from build123d import *

# Parameters (mm, degrees)
SKETCH2_W           = 81.6
SKETCH2_H           = 24
SKETCH2_W_2         = 77.6
SKETCH2_H_2         = 20
BOSS_EXTRUDE1_DEPTH = 7.7
SKETCH3_W           = 77.6
SKETCH3_H           = 20
BOSS_EXTRUDE2_DEPTH = 2
SKETCH4_W           = 16.3
SKETCH4_H           = 13
CUT_EXTRUDE1_DEPTH  = 8.7
CUT_EXTRUDE2_REACH  = 83.6
SKETCH5_W           = 8
SKETCH5_H           = 6.8
SKETCH6_W           = 16.3
SKETCH6_H           = 2.5
SKETCH6_W_2         = 5
BOSS_EXTRUDE3_DEPTH = 4.9
SKETCH8_R           = 2.5
CUT_EXTRUDE3_DEPTH  = 2
SKETCH9_R           = 1.4
BOSS_EXTRUDE4_DEPTH = 2
SKETCH10_R          = 1.4
BOSS_EXTRUDE5_DEPTH = 2.9
CHAMFER1_SIZE       = 1.5
SKETCH11_W          = 1.1
SKETCH11_H          = 1.1
CUT_EXTRUDE4_DEPTH  = 25
LPATTERN1_COUNT     = 4
LPATTERN1_PITCH     = 2.2
LPATTERN2_COUNT     = 4
LPATTERN2_PITCH     = 2.2
SKETCH12_W          = 1.1
SKETCH12_H          = 1.1
CUT_EXTRUDE5_DEPTH  = 28
LPATTERN3_COUNT     = 3
LPATTERN3_PITCH     = 2.2
LPATTERN4_COUNT     = 3
LPATTERN4_PITCH     = 2.2


with BuildPart() as part:
    # Sketch2 → Boss-Extrude1 (new body)
    with BuildSketch(Plane(origin=(0, 0, 0), x_dir=(1, 0, 0), z_dir=(0, 1, 0))):
        Rectangle(SKETCH2_W, SKETCH2_H)
        Rectangle(SKETCH2_W_2, SKETCH2_H_2, mode=Mode.SUBTRACT)
    extrude(amount=BOSS_EXTRUDE1_DEPTH)

    # Sketch3 → Boss-Extrude2 (add)
    with BuildSketch(Plane(origin=(0, 7.7, 0), x_dir=(1, 0, 0), z_dir=(0, 1, 0))):
        Rectangle(SKETCH3_W, SKETCH3_H)
    extrude(amount=-BOSS_EXTRUDE2_DEPTH)

    # Sketch4 → Cut-Extrude1 (cut, through all)
    with BuildSketch(Plane(origin=(0, 7.7, 0), x_dir=(1, 0, 0), z_dir=(0, 1, 0))):
        with Locations((-26.8, 0)):
            Rectangle(SKETCH4_W, SKETCH4_H)
    extrude(amount=-CUT_EXTRUDE1_DEPTH, mode=Mode.SUBTRACT)

    # Sketch5 → Cut-Extrude2 (cut, up to next)
    with BuildSketch(Plane(origin=(40.8, 0, 0), x_dir=(0, 0, -1), z_dir=(1, 0, 0)), mode=Mode.PRIVATE) as cut_extrude2_sk1:
        Rectangle(SKETCH5_W, SKETCH5_H)
    cut_extrude2_tool1 = extrude(cut_extrude2_sk1.sketch, amount=-CUT_EXTRUDE2_REACH, mode=Mode.PRIVATE) & part.part
    add(cut_extrude2_tool1.solids().sort_by_distance((40.8, 0, 0))[0], mode=Mode.SUBTRACT)

    # Sketch6 → Boss-Extrude3 (add)
    with BuildSketch(Plane.XZ.offset(-5.7)):
        with Locations((-26.8, 8.75)):
            Rectangle(SKETCH6_W, SKETCH6_H)
        with Locations((-26.8, -8.75)):
            Rectangle(SKETCH6_W, SKETCH6_H)
        with Locations((30.65, 8.75)):
            Rectangle(SKETCH6_W, SKETCH6_H)
        with Locations((36.3, -8.75)):
            Rectangle(SKETCH6_W_2, SKETCH6_H)
    extrude(amount=BOSS_EXTRUDE3_DEPTH)

    # Sketch8 → Cut-Extrude3 (cut)
    with BuildSketch(Plane(origin=(0, 7.7, 0), x_dir=(1, 0, 0), z_dir=(0, 1, 0))):
        with Locations((-7.9, 7.6)):
            Circle(SKETCH8_R)
        with Locations((-7.9, -7.4)):
            Circle(SKETCH8_R)
    extrude(amount=-CUT_EXTRUDE3_DEPTH, mode=Mode.SUBTRACT)

    # Sketch9 → Boss-Extrude4 (add)
    with BuildSketch(Plane.XZ.offset(-5.7)):
        Polygon((-4.15, 4.8), (-4.15, 10), (-11.65, 10), (-11.65, 4.8), (-11.65, -5.2), (-11.65, -10), (-4.15, -10), (-4.15, -5.2), align=None)
        with Locations((-7.9, 7.4)):
            Circle(SKETCH9_R, mode=Mode.SUBTRACT)
        with Locations((-7.9, -7.6)):
            Circle(SKETCH9_R, mode=Mode.SUBTRACT)
    extrude(amount=BOSS_EXTRUDE4_DEPTH)

    # Sketch10 → Boss-Extrude5 (add)
    with BuildSketch(Plane.XZ.offset(-3.7)):
        with BuildLine():
            Line((-10.3, 7.4), (-10.3, 10))
            Line((-10.3, 10), (-5.5, 10))
            Line((-5.5, 10), (-5.5, 7.4))
            ThreePointArc((-5.5, 7.4), (-7.9, 5), (-10.3, 7.4))
        make_face()
        with Locations((-7.9, 7.4)):
            Circle(SKETCH10_R, mode=Mode.SUBTRACT)
        with BuildLine():
            Line((-10.3, -7.6), (-10.3, -10))
            Line((-10.3, -10), (-5.5, -10))
            Line((-5.5, -10), (-5.5, -7.6))
            ThreePointArc((-5.5, -7.6), (-7.9, -5.2), (-10.3, -7.6))
        make_face()
        with Locations((-7.9, -7.6)):
            Circle(SKETCH10_R, mode=Mode.SUBTRACT)
    extrude(amount=BOSS_EXTRUDE5_DEPTH)

    # Chamfer1
    chamfer1_edges = [part.edges().sort_by_distance(p)[0] for p in [
        (-18.65, 7.7, 0),
        (-26.8, 7.7, -6.5),
        (-34.95, 7.7, 0),
        (-26.8, 7.7, 6.5),
    ]]
    chamfer(chamfer1_edges, length=CHAMFER1_SIZE)

    # Sketch11 → Cut-Extrude4 (cut, through all)
    with BuildSketch(Plane.XY.offset(12)):
        with Locations((-26.8, 7.7)):
            Rectangle(SKETCH11_W, SKETCH11_H)
    cut_extrude4 = extrude(amount=-CUT_EXTRUDE4_DEPTH, mode=Mode.SUBTRACT)

    # LPattern1: Cut-Extrude4 ×4
    with Locations(*[(i * LPATTERN1_PITCH, 0, 0) for i in range(1, LPATTERN1_COUNT)]):
        add(cut_extrude4, mode=Mode.SUBTRACT)

    # LPattern2: Cut-Extrude4 ×4
    with Locations(*[(-i * LPATTERN2_PITCH, 0, 0) for i in range(1, LPATTERN2_COUNT)]):
        add(cut_extrude4, mode=Mode.SUBTRACT)

    # Sketch12 → Cut-Extrude5 (cut)
    with BuildSketch(Plane.ZY.offset(40.8)):
        with Locations((0, 7.7)):
            Rectangle(SKETCH12_W, SKETCH12_H)
    cut_extrude5 = extrude(amount=-CUT_EXTRUDE5_DEPTH, mode=Mode.SUBTRACT)

    # LPattern3: Cut-Extrude5 ×3
    with Locations(*[(0, 0, i * LPATTERN3_PITCH) for i in range(1, LPATTERN3_COUNT)]):
        add(cut_extrude5, mode=Mode.SUBTRACT)

    # LPattern4: Cut-Extrude5 ×3
    with Locations(*[(0, 0, -i * LPATTERN4_PITCH) for i in range(1, LPATTERN4_COUNT)]):
        add(cut_extrude5, mode=Mode.SUBTRACT)


solid = part.part
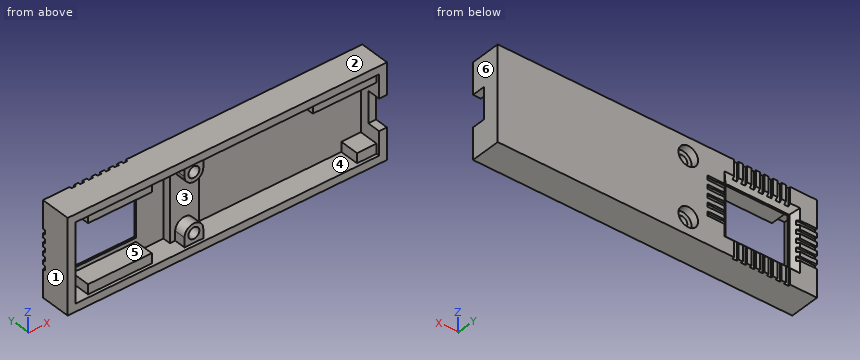
Design review of the part built by this model. Coordinates are the model's own, in mm. Face numbers are marked on the shaded views. A direction names the side the tool comes from. Coordinates: 2 decimals unless noted, no trailing zeros. Loops run counter-clockwise (first coordinate to the right, second up) from the corner with the lowest first, then second, coordinate; pieces in that order, holes last.
Item 1: Draft analysis for pull direction X (two halves, no side actions). For the marked faces 1, 2, 3 and 4, state which applies: pulls with the +X half, pulls with the -X half, needs draft (parallel to the pull), parting line crosses it, or undercut.
Completed:
face 1: pulls with the -X half
face 2: needs draft
face 3: undercut
face 4: undercut
Item 2: Add section C-C (x = 1). Write out the cut boundary in (y, z).
Completed:
outline: (0, -12) - (7.7, -12) - (7.7, 12) - (0, 12) - (0, 10) - (5.7, 10) - (5.7, -10) - (0, -10) - close
Item 3: Clearance check with flat-ended pins moving along their axes: pin 1 (0.6 mm diameter, centred on x = -20, z = -9.5, fed in from +Y); pin 2 (2 mm diameter, centred on x = -6.5, z = -1, fed in from -Y); pin 3 (6 mm diameter, centred on x = -29.5, z = -7.5, fed in from +Y). State where each tip first meets the part, or that it passes through.
Completed:
pin 1: stops at y = 7.15
pin 2: stops at y = 3.7
pin 3: stops at y = 7.7
Item 4: Add section B-B (x = -7.9). Write out the cut boundary in (y, z), and give its area (3 significant figures).
Completed:
outline: (0, -12) - (7.7, -12) - (7.7, -10.1) - (5.7, -10.1) - (5.7, -9) - (0.8, -9) - (0.8, -10) - (0, -10) - close; (0, 10) - (0.8, 10) - (0.8, 8.8) - (5.7, 8.8) - (5.7, 9.9) - (7.7, 9.9) - (7.7, 12) - (0, 12) - close; (0.8, -6.2) - (5.7, -6.2) - (5.7, -5.1) - (7.7, -5.1) - (7.7, 4.9) - (5.7, 4.9) - (5.7, 6) - (0.8, 6) - (0.8, 5) - (3.7, 5) - (3.7, -5.2) - (0.8, -5.2) - close
area: 91.8 mm2
Item 5: For the marked faces 5 and 6, list the 3-axis set-ups (+Z, -Z, +X, -X, +Y, -Y) from which the entire face can be reached by the end or side of a thin tool; tool diameter is ignored.
Completed:
face 5: -Y
face 6: +Z, -Z, +X, +Y, -Y
Item 6: Wall thickness on L1, parallel to X at y = 4, z = 1; L2, parallel to Z at x = -7.9, y = 4.65; L3, parallel to Z at x = -11, y = 2.25: over which ranges is each line inside the solid? List them lowest first.
Completed:
L1: x = -40.8 to -38.8, -11.65 to -4.15, 38.8 to 40.8
L2: z = -12 to -9, -6.2 to 6, 8.8 to 12
L3: z = -12 to -10, 10 to 12
Item 7: Add section A-A (y = 4.5). Write out the cut boundary in (x, z), and give its area (3 significant figures).
Completed:
outline: (-40.8, -12) - (40.8, -12) - (40.8, 12) - (-40.8, 12) - close; hole (-38.8, -10) - (-34.95, -10) - (-34.95, -7.5) - (-18.65, -7.5) - (-18.65, -10) - (-11.65, -10) - (-11.65, 10) - (-18.65, 10) - (-18.65, 7.5) - (-34.95, 7.5) - (-34.95, 10) - (-38.8, 10) - close; hole circle Ø2.8 at (-7.9, -7.6); hole circle Ø2.8 at (-7.9, 7.4); hole (-4.15, -10) - (33.8, -10) - (33.8, -7.5) - (38.8, -7.5) - (38.8, 7.5) - (22.5, 7.5) - (22.5, 10) - (-4.15, 10) - close
area: 679 mm2
